Geometry check sheet. Reference: the model listing, model coordinates, mm. Give positions to 0.01 mm unless a question says otherwise; leave off trailing zeros. Order: outer loops, then holes, each group sorted by start corner. A loop starts at its lowest first (then second) coordinate and runs counter-clockwise, first axis right, second up. Notation, with made-up numbers: M 42,17 L 63,17 A35 ccw 63,55 Z; hole C -0.75,68.25 d3. An arc over 180 degrees is marked long. Put each result on its own line as item: value. Start each with the question number.
Q1. Section check D-D on z = -3.5. Record the cut outline in (x, y).
Q2. Section check A-A on z = 12.5. Record the cut outline in (x, y).
Q3. Section check B-B on y = 2.05. Record the cut outline in (x, z), then the cut area to 3 significant figures.
Q4. Material ranges on L1, parallel to Z at x = -33, y = 3.7; L2, parallel to Z at x = -10, y = 0.9; L3, parallel to X at y = 0.8, z = -1.5, recorded low to high.
Q5. Go/stop test with a flat-tipped pin: pin 1 (2.5 mm diameter, centred on x = 25, y = 2.5, fed in from -Z). Record where the tip stops, or that it passes through.
Q6. Section check C-C on x = -35. Record the cut outline in (y, z), then the cut area to 3 significant figures.
```python
from build123d import *

# Parameters (mm, degrees)
SKETCH2_W           = 100
SKETCH2_H           = 50
BOSS_EXTRUDE1_DEPTH = 5
SKETCH3_W           = 10
SKETCH3_H           = 17.5
CUT_EXTRUDE1_DEPTH  = 7.5
CUT_EXTRUDE2_DEPTH  = 7.5
SKETCH5_W           = 50
SKETCH5_H           = 50
BOSS_EXTRUDE2_DEPTH = 5
CUT_EXTRUDE3_DEPTH  = 10
LPATTERN1_COUNT     = 2
LPATTERN1_PITCH     = 25


with BuildPart() as part:
    # Sketch2 → Boss-Extrude1 (new body)
    with BuildSketch(Plane(origin=(0, 0, 0), x_dir=(1, 0, 0), z_dir=(0, 1, 0))):
        Rectangle(SKETCH2_W, SKETCH2_H)
    extrude(amount=BOSS_EXTRUDE1_DEPTH)

    # Sketch3 → Cut-Extrude1 (cut)
    with BuildSketch(Plane(origin=(0, 5, 0), x_dir=(1, 0, 0), z_dir=(0, 1, 0))):
        with Locations((15, 0)):
            Rectangle(SKETCH3_W, SKETCH3_H)
    extrude(amount=-CUT_EXTRUDE1_DEPTH, mode=Mode.SUBTRACT)

    # Sketch4 → Cut-Extrude2 (cut)
    with BuildSketch(Plane(origin=(0, 5, 0), x_dir=(1, 0, 0), z_dir=(0, 1, 0))):
        with BuildLine():
            Line((-45, 15), (-15, 15))
            ThreePointArc((-15, 15), (-12.5, 12.5), (-15, 10))
            Line((-15, 10), (-45, 10))
            ThreePointArc((-45, 10), (-47.5, 12.5), (-45, 15))
        make_face()
        with BuildLine():
            Line((-45, -15), (-15, -15))
            ThreePointArc((-15, -15), (-12.5, -12.5), (-15, -10))
            Line((-15, -10), (-45, -10))
            ThreePointArc((-45, -10), (-47.5, -12.5), (-45, -15))
        make_face()
    extrude(amount=-CUT_EXTRUDE2_DEPTH, mode=Mode.SUBTRACT)

    # Sketch5 → Boss-Extrude2 (add)
    with BuildSketch(Plane(origin=(0, 5, 0), x_dir=(1, 0, 0), z_dir=(0, 1, 0))):
        with Locations((-25, 50)):
            Rectangle(SKETCH5_W, SKETCH5_H)
    extrude(amount=-BOSS_EXTRUDE2_DEPTH)

    # Sketch6 → Cut-Extrude3 (cut)
    with BuildSketch(Plane(origin=(0, 5, 0), x_dir=(1, 0, 0), z_dir=(0, 1, 0))):
        with BuildLine():
            Line((-45, 38.880259694), (-7.5, 38.880259694))
            ThreePointArc((-7.5, 38.880259694), (-5, 36.380259694), (-7.5, 33.880259694))
            Line((-7.5, 33.880259694), (-45, 33.880259694))
            ThreePointArc((-45, 33.880259694), (-47.5, 36.380259694), (-45, 38.880259694))
        make_face()
    cut_extrude3 = extrude(amount=-CUT_EXTRUDE3_DEPTH, mode=Mode.SUBTRACT)

    # LPattern1: Cut-Extrude3 ×2
    with Locations(*[(0, 0, -i * LPATTERN1_PITCH) for i in range(1, LPATTERN1_COUNT)]):
        add(cut_extrude3, mode=Mode.SUBTRACT)


solid = part.part
```
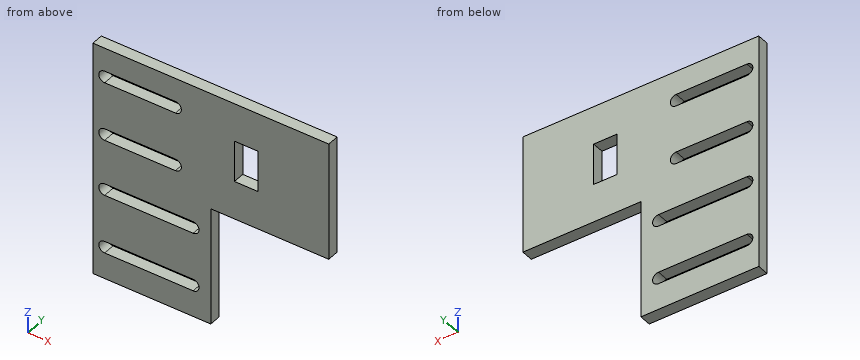
Results found:
1. outline: M -50,0 L 10,0 L 10,5 L -50,5 Z; M 20,0 L 50,0 L 50,5 L 20,5 Z
2. outline: M -50,0 L -47.5,0 L -47.5,5 L -50,5 Z; M -12.5,0 L 50,0 L 50,5 L -12.5,5 Z
3. outline: M -50,-75 L 0,-75 L 0,-25 L 50,-25 L 50,25 L -50,25 Z; hole M -45,-63.88 L -7.5,-63.88 A2.5 ccw -7.5,-58.88 L -45,-58.88 A2.5 ccw Z; hole M -45,-38.88 L -7.5,-38.88 A2.5 ccw -7.5,-33.88 L -45,-33.88 A2.5 ccw Z; hole M -45,-15 L -15,-15 A2.5 ccw -15,-10 L -45,-10 A2.5 ccw Z; hole M -45,10 L -15,10 A2.5 ccw -15,15 L -45,15 A2.5 ccw Z; hole M 10,-8.75 L 20,-8.75 L 20,8.75 L 10,8.75 Z
3. area: 6,570 mm^2
4. L1: z = -75 to -63.88, -58.88 to -38.88, -33.88 to -15, -10 to 10, 15 to 25
4. L2: z = -75 to -63.88, -58.88 to -38.88, -33.88 to 25
4. L3: x = -50 to 10, 20 to 50
5. pin 1: stops at z = -25
6. outline: M 0,-75 L 5,-75 L 5,-63.88 L 0,-63.88 Z; M 0,-58.88 L 5,-58.88 L 5,-38.88 L 0,-38.88 Z; M 0,-33.88 L 5,-33.88 L 5,-15 L 0,-15 Z; M 0,-10 L 5,-10 L 5,10 L 0,10 Z; M 0,15 L 5,15 L 5,25 L 0,25 Z
6. area: 400 mm^2
